The model under review builds one solid part; all positions refer to its coordinate system, in mm. A direction names the side the tool comes from. Give positions to 0.01 mm unless a question says otherwise; leave off trailing zeros. Write each loop counter-clockwise with the first axis right and the second up, starting at its lowest first coordinate (ties: lowest second). Pieces come first, ordered by that corner, then holes. Notation, with made-up numbers: M 50.5,16 L 91.5,16 A25 ccw 91.5,55 Z; hole C 9.25,3.25 d2. An arc over 180 degrees is marked long. Write each question's results on one line, items separated by ' | '. Start each with the question number.
from build123d import *

# Parameters (mm, degrees)
SKETCH2_R           = 2.55
BOSS_EXTRUDE1_DEPTH = 50
SKETCH6_W           = 35
SKETCH6_H           = 8
CUT_EXTRUDE3_DEPTH  = 31
CUT_EXTRUDE6_DEPTH  = 75
SKETCH9_R           = 5
BOSS_EXTRUDE2_DEPTH = 20
REVOLVE1_ANGLE      = 180
FILLET2_R           = 1


with BuildPart() as part:
    # Sketch2 → Boss-Extrude1 (new body)
    with BuildSketch(Plane.XY):
        with BuildLine():
            Line((0, 15), (100, 15))
            ThreePointArc((100, 15), (115, 0), (100, -15))
            Line((100, -15), (0, -15))
            Line((0, -15), (0, 15))
        make_face()
        with Locations((100, 0)):
            Circle(SKETCH2_R, mode=Mode.SUBTRACT)
    boss_extrude1 = extrude(amount=BOSS_EXTRUDE1_DEPTH)

    # Sketch6 → Cut-Extrude3 (cut, through all)
    with BuildSketch(Plane(origin=(0, 15, 0), x_dir=(1, 0, 0), z_dir=(0, 1, 0))):
        with Locations((97.5, -25)):
            Rectangle(SKETCH6_W, SKETCH6_H)
    cut_extrude3 = extrude(amount=-CUT_EXTRUDE3_DEPTH, mode=Mode.SUBTRACT)

    # Sketch7 → Cut-Extrude6 (cut)
    with BuildSketch(Plane.ZY):
        with BuildLine():
            Line((3, 15), (47, 15))
            ThreePointArc((47, 15), (25, -7), (3, 15))
        make_face()
    cut_extrude6 = extrude(amount=-CUT_EXTRUDE6_DEPTH, mode=Mode.SUBTRACT)

    # Mirror3: Boss-Extrude1, Cut-Extrude3, Cut-Extrude6 across plane
    add(boss_extrude1.mirror(Plane(origin=(0, -15, 50), x_dir=(0, 0, 1), z_dir=(-1, 0, 0))))
    add(cut_extrude3.mirror(Plane(origin=(0, -15, 50), x_dir=(0, 0, 1), z_dir=(-1, 0, 0))), mode=Mode.SUBTRACT)
    add(cut_extrude6.mirror(Plane(origin=(0, -15, 50), x_dir=(0, 0, 1), z_dir=(-1, 0, 0))), mode=Mode.SUBTRACT)

    # Sketch9 → Boss-Extrude2 (add)
    with BuildSketch(Plane.XY.offset(50)):
        Circle(SKETCH9_R)
    boss_extrude2 = extrude(amount=BOSS_EXTRUDE2_DEPTH)

    # Sketch12 → Revolve1 (revolve)
    with BuildSketch(Plane.XY.offset(70)):
        with BuildLine():
            Line((0, -5), (0, 5))
            ThreePointArc((0, 5), (5, 0), (0, -5))
        make_face()
    revolve1 = revolve(axis=Axis((0, -5, 70), (0, -1, 0)), revolution_arc=REVOLVE1_ANGLE)

    # Mirror4: Boss-Extrude2, Revolve1 across plane
    add(boss_extrude2.mirror(Plane(origin=(75, -7, 25), x_dir=(1, 0, 0), z_dir=(0, 0, 1))))
    add(revolve1.mirror(Plane(origin=(75, -7, 25), x_dir=(1, 0, 0), z_dir=(0, 0, 1))))

    # Fillet2
    fillet2_edges = [part.edges().sort_by_distance(p)[0] for p in [
        (-5, 0, 50),
        (-5, 0, 0),
    ]]
    fillet(fillet2_edges, radius=FILLET2_R)


solid = part.part
(1) Add section C-C (z = 25). State the section outline as (x, y) points, then the cut area to 3 significant figures.
(2) Add section D-D (y = 11). State the section outline as (x, z) points, then the cut area to 3 significant figures.
(3) Machinability: for faces 5 (the flat face through (97, 0, 21)), 6 (the cylindrical face through (-1, -7, 25)), 7 (the flat face through (-97, 0, 21)), 8 (the cylindrical face through (-1.08, -4.88, -10.37)), which of the approach directions +Z, -Z, +X, -X, +Y, -Y give a long, thin tool a straight path to every point of the face, cutting with its end or side? Answer none if there is none.
(4) Wall thickness on L1, parallel to Z at x = 85, y = -11.5; L2, parallel to Y at x = 100, z = 41.75; L3, parallel to X at y = 3.75, z = 28.5: over which ranges is each line inside the solid? List them lowest first.
(5) Clearance check with flat-ended pins moving along their axes: P1, Ø15, axis at x = 105.5, y = -4.5, coming from the -Z side; P2, Ø6.5, axis at x = -100, y = 0, coming from the +Z side; P3, Ø12, axis at y = 6.5, z = 22.5, coming from the -X side. State where each tip first meets the part, or that it passes through.
(6) Draft analysis for pull direction Y (two halves, no side actions). For faces 1 (the cylindrical face through (102.43, 0.77, 39.35)), 2 (the cylindrical face through (-1.08, -4.88, 60.37)), 3 (the cylindrical face through (-102.43, 0.77, 10.35)), 4 (the flat face through (-97, 0, 29)), state which applies: pulls with the +Y half, pulls with the -Y half, needs draft (parallel to the pull), parting line crosses it, or undercut.
(7) Add section A-A (x = 83.5). State the section outline as (y, z) points, then the cut area to 3 significant figures.
(8) Add section B-B (z = 11). State the section outline as (x, y) points.
Calculated:
1) outline: M -80,-15 L 80,-15 L 80,15 L 75,15 L 75,-7 L -75,-7 L -75,15 L -80,15 Z | area: 1,500 mm²
2) outline: M -110.2,0 L 110.2,0 L 110.2,21 L 80,21 L 80,29 L 110.2,29 L 110.2,50 L -110.2,50 L -110.2,29 L -80,29 L -80,21 L -110.2,21 Z; hole M -75,3.37 L 75,3.37 L 75,46.63 L -75,46.63 Z | area: 4,050 mm²
3) face 5: +X, +Y, -Y | face 6: +Y | face 7: -X, +Y, -Y | face 8: -Z
4) L1: z = 0 to 21, 29 to 50 | L2: y = -15 to -2.55, 2.55 to 15 | L3: x = -80 to -75, 75 to 80
5) P1: stops at z = 0 | P2: stops at z = 50 | P3: stops at x = -114.98
6) face 1: undercut | face 2: parting line crosses it | face 3: undercut | face 4: needs draft
7) outline: M -15,0 L 15,0 L 15,21 L -15,21 Z; M -15,29 L 15,29 L 15,50 L -15,50 Z | area: 1,260 mm²
8) outline: M -100,-15 L 100,-15 A15 ccw 100,15 L 75,15 L 75,-1.97 L -75,-1.97 L -75,15 L -100,15 A15 ccw Z; hole C -100,0 d5.1; hole C 100,0 d5.1
